```python
from build123d import *

# Parameters (mm, degrees)
SKETCH_2_R          = 1.5
CUT_EXTRUDE_1_DEPTH = 10


with BuildPart() as part:
    # Эскиз1 → Повернуть1 (revolve)
    with BuildSketch(Plane.XY, mode=Mode.PRIVATE) as revolve_1_sk:
        Polygon((-17, 0), (-17, 36.5), (-16, 37.5), (-14, 37.5), (-14, 35.5), (-11, 35.5), (-9, 33.5), (-7, 35.5), (-5, 35.5), (-5, 33.5), (-2.5, 33.5), (-2.5, 35.5), (-0.5, 35.5), (0, 35), (0, 0), align=None)
    revolve(revolve_1_sk.sketch.rotate(Axis((0, 0, 0), (1, 0, 0)), 90), axis=Axis((0, 0, 0), (1, 0, 0)))

    # Эскиз2 → Вырез-Вытянуть1 (cut)
    with BuildSketch(Plane(origin=(0, 0, 0), x_dir=(0, 0, -1), z_dir=(1, 0, 0))):
        with Locations((20.784609691, -12)):
            Circle(SKETCH_2_R)
        with Locations((0, 24)):
            Circle(SKETCH_2_R)
        with Locations((-20.784609691, -12)):
            Circle(SKETCH_2_R)
    extrude(amount=-CUT_EXTRUDE_1_DEPTH, mode=Mode.SUBTRACT)


solid = part.part
```
Could you check a few things on this model? Use its own coordinates, in mm. A direction names the side the tool comes from. Give positions to 0.01 mm unless a question says otherwise; leave off trailing zeros. Loops run counter-clockwise (first coordinate to the right, second up) from the corner with the lowest first, then second, coordinate; pieces in that order, holes last. Notation, with made-up numbers: (-5, -16.75) - (44, -16.75) arc R17 ccw to (44, 12.25) - close; hole circle Ø2 at (-13, -34). An arc over 180 degrees is marked (long way). Answer in a Markdown table with one row per item. Add a question column.
Q1. Please list where these lines run through material, in increasing order: L1, parallel to Y at x = -4, z = 0; L2, parallel to X at y = -15, z = 31; L3, parallel to Y at x = -5.25, z = 0. Write a range as from..to.
Q2. We'd pull the mould along Z, two halves only. Please class faces 1 (the face through (-14.99, 33.27, 17.3)), 2 (the face through (-4.9, -11.5, -22.2)), 3 (the face through (-14, 33, 14)): +Z half, -Z half, draft (parallel to the pull), parting line (faces both ways), or undercut.
Q3. If we section it at B-B (y = 0): List the corners of the cut face in (x, z) for me.
Q4. Which directions (+Z, -Z, +X, -X, +Y, -Y) give clear straight access to the entire face, cutting with the end or side of a thin tool? Please do faces 4 (the face through (-4.93, -11.934, 22.283)), 5 (the face through (-17, -1, 1)), 6 (the face through (-3.7, 29.7, 15.5)).
Q5. For pin 1 (6 mm diameter, centred on x = -7, z = -26.5, fed in from -Y); pin 2 (1 mm diameter, centred on x = -14, y = -20, fed in from +Z); pin 3 (1 mm diameter, centred on x = -7, z = 13, fed in from +Y), each with a flat end and sliding along its axis, tell me the tip position at first contact or that it passes through.
Q6. If we section it at C-C (x = -1.5): List the corners of the cut face in (y, z) for me.
The answers:
| question | item | result |
|---|---|---|
| 1 | L1 | y = -33.5..22.5, 25.5..33.5 |
| 1 | L2 | x = -17..-9.94, -8.06..-5, -2.5..0 |
| 1 | L3 | y = -35.5..22.5, 25.5..35.5 |
| 2 | face 1 | parting line |
| 2 | face 2 | undercut |
| 2 | face 3 | draft |
| 3 | outline | (-17, -36.5) - (-16, -37.5) - (-14, -37.5) - (-14, -35.5) - (-11, -35.5) - (-9, -33.5) - (-7, -35.5) - (-5, -35.5) - (-5, -33.5) - (-2.5, -33.5) - (-2.5, -35.5) - (-0.5, -35.5) - (0, -35) - (0, 35) - (-0.5, 35.5) - (-2.5, 35.5) - (-2.5, 33.5) - (-5, 33.5) - (-5, 35.5) - (-7, 35.5) - (-9, 33.5) - (-11, 35.5) - (-14, 35.5) - (-14, 37.5) - (-16, 37.5) - (-17, 36.5) - close |
| 4 | face 4 | +X |
| 4 | face 5 | +Z, -Z, -X, +Y, -Y |
| 4 | face 6 | none |
| 5 | pin 1 | stops at y = -26.61 |
| 5 | pin 2 | stops at z = 32.03 |
| 5 | pin 3 | stops at y = 33.23 |
| 6 | outline | circle Ø71 at (0, 0); hole circle Ø3 at (-12, -20.78); hole circle Ø3 at (-12, 20.78); hole circle Ø3 at (24, 0) |
